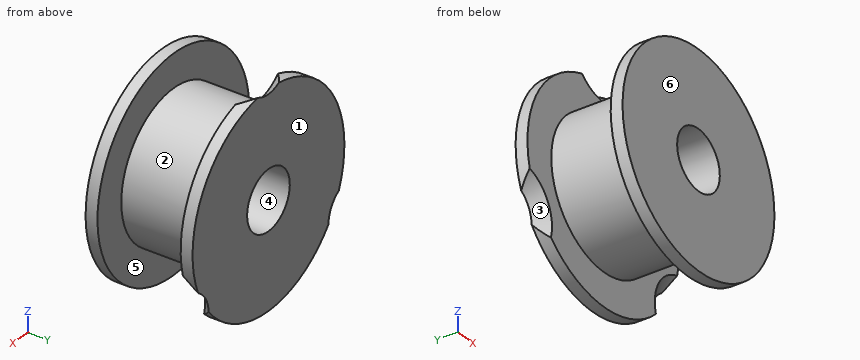
```python
from build123d import *

# Parameters (mm, degrees)
ENL_V_MAT_EXTRU_1_REACH = 16.914
ESQUISSE2_R             = 2.5
CHANFREIN1_SIZE         = 1


with BuildPart() as part:
    # Esquisse1 → Révolution1 (revolve)
    with BuildSketch(Plane.XY, mode=Mode.PRIVATE) as r_volution1_sk:
        Polygon((2.5, 0), (8.9, 0), (8.9, 1), (6.11, 1), (6.11, 8), (8.9, 8), (8.9, 9), (2.5, 9), align=None)
    revolve(r_volution1_sk.sketch.rotate(Axis((0, 0, 0), (0, 1, 0)), 90), axis=Axis((0, 0, 0), (0, 1, 0)))

    # Esquisse2 → Enlèv. mat.-Extru.1 (cut, up to next)
    with BuildSketch(Plane.XZ.offset(-8), mode=Mode.PRIVATE) as enl_v_mat_extru_1_sk1:
        with Locations((0, 11)):
            Circle(ESQUISSE2_R)
    enl_v_mat_extru_1_tool1 = extrude(enl_v_mat_extru_1_sk1.sketch, amount=-ENL_V_MAT_EXTRU_1_REACH, mode=Mode.PRIVATE) & part.part
    # Esquisse2 → Enlèv. mat.-Extru.1 (cut, up to next)
    with BuildSketch(Plane.XZ.offset(-8), mode=Mode.PRIVATE) as enl_v_mat_extru_1_sk2:
        with Locations((9.526279442, -5.5)):
            Circle(ESQUISSE2_R)
    enl_v_mat_extru_1_tool2 = extrude(enl_v_mat_extru_1_sk2.sketch, amount=-ENL_V_MAT_EXTRU_1_REACH, mode=Mode.PRIVATE) & part.part
    # Esquisse2 → Enlèv. mat.-Extru.1 (cut, up to next)
    with BuildSketch(Plane.XZ.offset(-8), mode=Mode.PRIVATE) as enl_v_mat_extru_1_sk3:
        with Locations((-9.526279442, -5.5)):
            Circle(ESQUISSE2_R)
    enl_v_mat_extru_1_tool3 = extrude(enl_v_mat_extru_1_sk3.sketch, amount=-ENL_V_MAT_EXTRU_1_REACH, mode=Mode.PRIVATE) & part.part
    add(enl_v_mat_extru_1_tool1.solids().sort_by_distance((0, 8, 11))[0], mode=Mode.SUBTRACT)
    add(enl_v_mat_extru_1_tool2.solids().sort_by_distance((9.526279, 8, -5.5))[0], mode=Mode.SUBTRACT)
    add(enl_v_mat_extru_1_tool3.solids().sort_by_distance((-9.526279, 8, -5.5))[0], mode=Mode.SUBTRACT)

    # Chanfrein1
    chanfrein1_edges = [part.edges().sort_by_distance(p)[0] for p in [
        (7.361215932, 8, -4.25),
        (0, 8, 8.5),
        (-7.361215932, 8, -4.25),
    ]]
    chamfer(chanfrein1_edges, length=CHANFREIN1_SIZE - 0.0001)  # a hair under: the kernel refuses the full size


solid = part.part
```
Could you check a few things on this model? Use its own coordinates, in mm. Face numbers are marked on the shaded views. A direction names the side the tool comes from. Coordinates: 2 decimals unless noted, no trailing zeros. Write each loop counter-clockwise with the first axis right and the second up, starting at its lowest first coordinate (ties: lowest second). Pieces come first, ordered by that corner, then holes. Notation, with made-up numbers: M 9.5,32.5 L 62.5,32.5 A15 cw 62.5,41.5 Z; hole C -12.75,44.5 d11. An arc over 180 degrees is marked long. Answer as CSV lines item,"result". Start each with the question number.
1) For the marked faces 1 and 2, which set-ups out of +Z, -Z, +X, -X, +Y, -Y let a thin tool reach every point of the face, with its end or its side?
2) I want a section at B-B, the plane z = 0. Please give me the cut outline in (x, y).
3) I want a section at C-C, the plane y = 5.5. Please give me the cut outline in (x, z), and give its area (3 significant figures).
4) We'd pull the mould along Y, two halves only. Please class the marked faces 3, 4, 5 and 6: +Y half, -Y half, draft (parallel to the pull), parting line (faces both ways), or undercut.
5) For P1, Ø1.5, axis at y = 4, z = 7, coming from the -X side; P2, Ø2, axis at x = 6.5, y = 3.5, coming from the -Z side; P3, Ø4, axis at y = 3.5, z = 1, coming from the +X side, each with a flat end and sliding along its axis, tell me the tip position at first contact or that it passes through.
6) I want a section at D-D, the plane z = 5.5. Please give me the cut outline in (x, y).
7) Please list where these lines run through material, in increasing order: line 1 (Y direction, x = -4.5, z = -4.75); line 2 (X direction, y = 2.75, z = 0); line 3 (X direction, y = 8.25, z = 1.5). Write a range as from..to.
Data:
1,face 1,"+Z, -Z, +X, -X, +Y"
1,face 2,"none"
2,outline,"M -8.9,0 L -2.5,0 L -2.5,9 L -8.9,9 L -8.9,8 L -6.11,8 L -6.11,1 L -8.9,1 Z; M 2.5,0 L 8.9,0 L 8.9,1 L 6.11,1 L 6.11,8 L 8.9,8 L 8.9,9 L 2.5,9 Z"
3,outline,"C 0,0 d12.22; hole C 0,0 d5"
3,area,"97.6 mm^2"
4,face 3,"undercut"
4,face 4,"draft"
4,face 5,"undercut"
4,face 6,"-Y half"
5,P1,"passes through"
5,P2,"stops at z = -2.66"
5,P3,"stops at x = 6.11"
6,outline,"M -7,0 L 7,0 L 7,1 L 2.66,1 L 2.66,8 L 7,8 L 7,9 L -7,9 L -7,8 L -2.66,8 L -2.66,1 L -7,1 Z"
7,line 1,"y = 0..1, 8..9"
7,line 2,"x = -6.11..-2.5, 2.5..6.11"
7,line 3,"x = -8.77..-2, 2..8.77"
